Work out the finished part from the listing and answer in its coordinate system (mm). A direction names the side the tool comes from. Give positions to 0.01 mm unless a question says otherwise; leave off trailing zeros. Order: outer loops, then holes, each group sorted by start corner. A loop starts at its lowest first (then second) coordinate and runs counter-clockwise, first axis right, second up. Notation, with made-up numbers: M 41,39 L 79,39 A17 ccw 79,47 Z; hole C 80.25,0.5 d7. An arc over 180 degrees is marked long. One line per item, written item: value.
from build123d import *

# Parameters (mm, degrees)
SKETCH1_W           = 286
SKETCH1_H           = 242
BOSS_EXTRUDE1_DEPTH = 43
FILLET1_R           = 33
SHELL1_T            = -3
BOSS_EXTRUDE2_DEPTH = 10
FILLET2_R           = 5
CUT_EXTRUDE2_DEPTH  = 245.651256349
FILLET3_R           = 2
BOSS_EXTRUDE3_REACH = 314.753
SKETCH5_W           = 40
SKETCH5_H           = 18
BOSS_EXTRUDE4_REACH = 314.753


with BuildPart() as part:
    # Sketch1 → Boss-Extrude1 (new body)
    with BuildSketch(Plane(origin=(0, 0, 0), x_dir=(1, 0, 0), z_dir=(0, 1, 0))):
        with Locations((24.44, -38.06)):
            Rectangle(SKETCH1_W, SKETCH1_H)
    extrude(amount=BOSS_EXTRUDE1_DEPTH)

    # Fillet1
    fillet1_edges = [part.edges().sort_by_distance(p)[0] for p in [
        (24.44, 43, 159.06),
        (-118.56, 43, 38.06),
        (24.44, 43, -82.94),
        (-118.56, 21.5, -82.94),
        (-118.56, 21.5, 159.06),
        (167.44, 21.5, 159.06),
        (167.44, 21.5, -82.94),
        (167.44, 43, 38.06),
    ]]
    fillet(fillet1_edges, radius=FILLET1_R)

    # Shell1
    shell1_openings = [part.faces().sort_by_distance(p)[0] for p in [
        (24.44, 0, 38.06),
    ]]
    offset(amount=SHELL1_T, openings=shell1_openings, kind=Kind.INTERSECTION)

    # Sketch2 → Boss-Extrude2 (add)
    with BuildSketch(Plane.XZ):
        with BuildLine():
            Line((-85.56, 166.06), (134.44, 166.06))
            ThreePointArc((134.44, 166.06), (162.724271247, 154.344271247), (174.44, 126.06))
            Line((174.44, 126.06), (174.44, -49.94))
            ThreePointArc((174.44, -49.94), (162.724271247, -78.224271247), (134.44, -89.94))
            Line((134.44, -89.94), (-85.56, -89.94))
            ThreePointArc((-85.56, -89.94), (-113.844271247, -78.224271247), (-125.56, -49.94))
            Line((-125.56, -49.94), (-125.56, 126.06))
            ThreePointArc((-125.56, 126.06), (-113.844271247, 154.344271247), (-85.56, 166.06))
        make_face()
        with BuildLine():
            Line((-85.56, 159.06), (134.44, 159.06))
            ThreePointArc((134.44, 159.06), (157.774523779, 149.394523779), (167.44, 126.06))
            Line((167.44, 126.06), (167.44, -49.94))
            ThreePointArc((167.44, -49.94), (157.774523779, -73.274523779), (134.44, -82.94))
            Line((134.44, -82.94), (-85.56, -82.94))
            ThreePointArc((-85.56, -82.94), (-108.894523779, -73.274523779), (-118.56, -49.94))
            Line((-118.56, -49.94), (-118.56, 126.06))
            ThreePointArc((-118.56, 126.06), (-108.894523779, 149.394523779), (-85.56, 159.06))
        make_face(mode=Mode.SUBTRACT)
    extrude(amount=-BOSS_EXTRUDE2_DEPTH)

    # Fillet2
    fillet2_edges = [part.edges().sort_by_distance(p)[0] for p in [
        (162.724271247, 10, -78.224271247),
        (24.44, 10, -89.94),
        (-113.844271247, 10, -78.224271247),
        (-125.56, 10, 38.06),
        (-113.844271247, 10, 154.344271247),
        (24.44, 10, 166.06),
        (162.724271247, 10, 154.344271247),
        (174.44, 10, 38.06),
    ]]
    fillet(fillet2_edges, radius=FILLET2_R)

    # Sketch4 → Cut-Extrude2 (cut, through all)
    with BuildSketch(Plane(origin=(0, 43, 0), x_dir=(1, 0, 0), z_dir=(0, 1, 0))):
        with BuildLine():
            Line((-23.684825583, 14.14), (72.564825583, 14.14))
            ThreePointArc((72.564825583, 14.14), (80.172419453, 10.630340169), (82.44, 2.564903101))
            Line((82.44, 2.564903101), (76.315174417, -35.835096899))
            ThreePointArc((76.315174417, -35.835096899), (72.930340169, -41.86759387), (66.44, -44.26))
            Line((66.44, -44.26), (-17.56, -44.26))
            ThreePointArc((-17.56, -44.26), (-24.050340169, -41.86759387), (-27.435174417, -35.835096899))
            Line((-27.435174417, -35.835096899), (-33.56, 2.564903101))
            ThreePointArc((-33.56, 2.564903101), (-31.292419453, 10.630340169), (-23.684825583, 14.14))
        make_face()
    extrude(amount=-CUT_EXTRUDE2_DEPTH, mode=Mode.SUBTRACT)

    # Fillet3
    fillet3_edges = [part.edges().sort_by_distance(p)[0] for p in [
        (-24.050340169, 43, 41.86759387),
        (24.44, 43, 44.26),
        (72.930340169, 43, 41.86759387),
        (79.377587208, 43, 16.635096899),
        (80.172419453, 43, -10.630340169),
        (24.44, 43, -14.14),
        (-31.292419453, 43, -10.630340169),
        (-30.497587208, 43, 16.635096899),
    ]]
    fillet(fillet3_edges, radius=FILLET3_R)

    # Sketch5 → Boss-Extrude3 (add, up to next)
    with BuildSketch(Plane(origin=(0, 0, -89.94), x_dir=(-1, 0, 0), z_dir=(0, 0, -1)), mode=Mode.PRIVATE) as boss_extrude3_sk1:
        with Locations((-94.44, 9)):
            Rectangle(SKETCH5_W, SKETCH5_H)
    boss_extrude3_tool1 = extrude(boss_extrude3_sk1.sketch, amount=-BOSS_EXTRUDE3_REACH, mode=Mode.PRIVATE) - part.part
    # Sketch5 → Boss-Extrude3 (add, up to next)
    with BuildSketch(Plane(origin=(0, 0, -89.94), x_dir=(-1, 0, 0), z_dir=(0, 0, -1)), mode=Mode.PRIVATE) as boss_extrude3_sk2:
        with Locations((45.56, 9)):
            Rectangle(SKETCH5_W, SKETCH5_H)
    boss_extrude3_tool2 = extrude(boss_extrude3_sk2.sketch, amount=-BOSS_EXTRUDE3_REACH, mode=Mode.PRIVATE) - part.part
    add(boss_extrude3_tool1.solids().sort_by_distance((94.44, 9, -89.94))[0])
    add(boss_extrude3_tool2.solids().sort_by_distance((-45.56, 9, -89.94))[0])

    # Sketch6 → Boss-Extrude4 (add, up to next)
    with BuildSketch(Plane.XY.offset(166.06), mode=Mode.PRIVATE) as boss_extrude4_sk1:
        with BuildLine():
            Line((-63.56, 5), (-27.56, 5))
            Line((-27.56, 5), (-27.56, 19))
            ThreePointArc((-27.56, 19), (-45.56, 25), (-63.56, 19))
            Line((-63.56, 19), (-63.56, 5))
        make_face()
    boss_extrude4_tool1 = extrude(boss_extrude4_sk1.sketch, amount=-BOSS_EXTRUDE4_REACH, mode=Mode.PRIVATE) - part.part
    # Sketch6 → Boss-Extrude4 (add, up to next)
    with BuildSketch(Plane.XY.offset(166.06), mode=Mode.PRIVATE) as boss_extrude4_sk2:
        with BuildLine():
            ThreePointArc((112.44, 19), (94.44, 25), (76.44, 19))
            Line((76.44, 19), (76.44, 5))
            Line((76.44, 5), (112.44, 5))
            Line((112.44, 5), (112.44, 19))
        make_face()
    boss_extrude4_tool2 = extrude(boss_extrude4_sk2.sketch, amount=-BOSS_EXTRUDE4_REACH, mode=Mode.PRIVATE) - part.part
    add(boss_extrude4_tool1.solids().sort_by_distance((-45.56, 14.129204, 166.06))[0])
    add(boss_extrude4_tool2.solids().sort_by_distance((94.44, 14.129204, 166.06))[0])


solid = part.part
(1) Find the intervals of material crossed by probe 1 along Z at (x, y) = (22, 3.5); probe 2 along X at (y, z) = (11, 74.5); probe 3 along X at (y, z) = (5, 66), in increasing order. Write a range as from..to.
Findings:
probe 1: z = -89.94..-79.94, 156.06..166.06
probe 2: x = -118.54..-115.54, 164.42..167.42
probe 3: x = -125.56..-115.56, 164.44..174.44
(2) Which of the six approach directions +Z, -Z, +X, -X, +Y, -Y give full straight-line access (tool end or side, diameter ignored) to faces 4 (the cylindrical face through (94.7, 25, 160.8)), 5 (the flat face through (-65.56, 14, -87)), 6 (the cylindrical face through (155.885, 5.07, -70.919)), 7 (the flat face through (74.44, 14, -87))?
Findings:
face 4: +Z, +Y
face 5: -Z, -X, +Y
face 6: -Y
face 7: -Z, +Y
(3) Given P1, Ø4, axis at y = 13, z = 163.5, coming from the +X side; P2, Ø6.5, axis at y = 9.5, z = -86, coming from the -X side; P3, Ø10, axis at y = 20.5, z = 11, coming from the +X side, each flat-ended and moving along its own axis, determine where each tip first touches the part or whether it passes through.
Findings:
P1: stops at x = 112.44
P2: stops at x = -106.18
P3: stops at x = 166.98
(4) Section D-D, the plane x = -76 is taken. Give the vertices of the cut face in (y, z).
Findings:
outline: M 0,-89.94 L 5,-89.94 A5 ccw 10,-84.94 L 10,-82.94 A33 ccw 43,-49.94 L 43,126.06 A33 ccw 10,159.06 L 10,161.06 A5 ccw 5,166.06 L 0,166.06 L 0,156.06 L 10,156.06 A30 cw 40,126.06 L 40,-49.94 A30 cw 10,-79.94 L 0,-79.94 Z
(5) Determine the mould class of faces 1 (the flat face through (95, 18, -86)), 2 (the cylindrical face through (163.034, 2.465, -77.912)), 3 (the cylindrical face through (-107.005, 5.07, 147.039)) for opening direction Z: pulls with the +Z half, pulls with the -Z half, needs draft (parallel to the pull), parting line crosses it, or undercut.
Findings:
face 1: needs draft
face 2: pulls with the -Z half
face 3: undercut
(6) Section C-C, the plane y = 32.5 is taken. Give the vertices of the cut face in (x, z).
Findings:
outline: M -109.7,-49.94 A24.14 ccw -85.56,-74.08 L 134.44,-74.08 A24.14 ccw 158.58,-49.94 L 158.58,126.06 A24.14 ccw 134.44,150.2 L -85.56,150.2 A24.14 ccw -109.7,126.06 Z; hole M -105.4,-49.94 A19.84 ccw -85.56,-69.78 L 134.44,-69.78 A19.84 ccw 154.28,-49.94 L 154.28,126.06 A19.84 ccw 134.44,145.9 L -85.56,145.9 A19.84 ccw -105.4,126.06 Z
(7) Section A-A, the plane x = 59 is taken. Give the vertices of the cut face in (y, z).
Findings:
outline: M 0,-89.94 L 5,-89.94 A5 ccw 10,-84.94 L 10,-82.94 A33 ccw 43,-49.94 L 43,-16.14 A2 ccw 41,-14.14 L 40,-14.14 L 40,-49.94 A30 cw 10,-79.94 L 0,-79.94 Z; M 0,156.06 L 10,156.06 A30 cw 40,126.06 L 40,44.26 L 41,44.26 A2 ccw 43,46.26 L 43,126.06 A33 ccw 10,159.06 L 10,161.06 A5 ccw 5,166.06 L 0,166.06 Z
(8) Section B-B, the plane z = 59 is taken. Give the vertices of the cut face in (x, y).
Findings:
outline: M -125.56,0 L -115.56,0 L -115.56,10 A30 cw -85.56,40 L 134.44,40 A30 cw 164.44,10 L 164.44,0 L 174.44,0 L 174.44,5 A5 ccw 169.44,10 L 167.44,10 A33 ccw 134.44,43 L -85.56,43 A33 ccw -118.56,10 L -120.56,10 A5 ccw -125.56,5 Z
